Read the model definition and answer for the solid it produces. Units are mm, in the model's axes. A direction names the side the tool comes from. Round coordinates to 2 decimals unless told otherwise and drop trailing zeros. Write each loop counter-clockwise with the first axis right and the second up, starting at its lowest first coordinate (ties: lowest second). Pieces come first, ordered by that corner, then holes. Notation, with made-up numbers: M -3.75,86 L 36.25,86 A26 cw 36.25,113 Z; hole C 34.5,1.25 d2. An arc over 180 degrees is marked long. Use one line per item in the form item = value. Start each with the question number.
```python
from build123d import *

# Parameters (mm, degrees)
BOSS_EXTRUDE1_START         = -15
BOSS_EXTRUDE1_DEPTH         = 30
BOSS_EXTRUDE1_START_2       = -12.7
BOSS_EXTRUDE1_2_OUTLINE_W   = 10
BOSS_EXTRUDE1_2_OUTLINE_H   = 5.949524979
BOSS_EXTRUDE1_2_DEPTH       = 25.4
BOSS_EXTRUDE1_3_OUTLINE_R   = 15
BOSS_EXTRUDE1_3_OUTLINE_R_2 = 4.55
BOSS_EXTRUDE1_3_DEPTH       = 19.994560744
SKETCH4_W                   = 3.6
SKETCH4_H                   = 22.4
CUT_EXTRUDE1_DEPTH          = 6
BOSS_EXTRUDE2_REACH         = 73.536
BOSS_EXTRUDE2_END_RADIUS    = 119.634966004
SKETCH9_R                   = 6.57997386
SKETCH9_R_2                 = 3.45
SKETCH10_W                  = 5.949524979
SKETCH10_H                  = 2.3
BOSS_EXTRUDE3_DEPTH         = 10
SKETCH11_W                  = 5.949524979
SKETCH11_H                  = 30
BOSS_EXTRUDE4_DEPTH         = 10
SKETCH13_W                  = 3.6
SKETCH13_H                  = 22.4
CUT_EXTRUDE2_DEPTH          = 10
CUT_EXTRUDE3_DEPTH          = 5


with BuildPart() as part:
    # Boss-Extrude1: read off the stored shape, not the designer's step
    # Boss-Extrude1 outline → Boss-Extrude1 (new body)
    with BuildSketch(Plane(origin=(0, 0, 0), x_dir=(1, 0, 0), z_dir=(0, 1, 0)).offset(BOSS_EXTRUDE1_START)):
        with BuildLine():
            Line((-50, -30), (-50, -35.949524979))
            ThreePointArc((-50, -35.949524979), (-25.592440765, -27.769436157), (0, -25))
            ThreePointArc((0, -25), (25.592440765, -27.769436157), (50, -35.949524979))
            Line((50, -35.949524979), (50, -30))
            ThreePointArc((50, -30), (27.810549479, -22.327809439), (4.550000287, -19.13702996))
            ThreePointArc((4.550000287, -19.13702996), (2.275411741, -19.072115713), (0, -19.050475021))
            ThreePointArc((0, -19.050475021), (-25.592440765, -21.819911178), (-50, -30))
        make_face()
    extrude(amount=BOSS_EXTRUDE1_DEPTH)

    # Boss-Extrude1 2 outline → Boss-Extrude1 2 (add)
    with BuildSketch(Plane(origin=(0, 0, 0), x_dir=(1, 0, 0), z_dir=(0, 1, 0)).offset(BOSS_EXTRUDE1_START_2)):
        with Locations((-55, -32.97476249)):
            Rectangle(BOSS_EXTRUDE1_2_OUTLINE_W, BOSS_EXTRUDE1_2_OUTLINE_H)
    extrude(amount=BOSS_EXTRUDE1_2_DEPTH)

    # Boss-Extrude1 3 outline → Boss-Extrude1 3 (add)
    with BuildSketch(Plane.XY):
        Circle(BOSS_EXTRUDE1_3_OUTLINE_R)
        Circle(BOSS_EXTRUDE1_3_OUTLINE_R_2, mode=Mode.SUBTRACT)
    extrude(amount=BOSS_EXTRUDE1_3_DEPTH)

    # Sketch4 → Cut-Extrude1 (cut)
    with BuildSketch(Plane.XY.offset(35.949524979)):
        with Locations((-53, 0)):
            Rectangle(SKETCH4_W, SKETCH4_H)
    extrude(amount=-CUT_EXTRUDE1_DEPTH, mode=Mode.SUBTRACT)

    # Boss-Extrude2: up to this cylinder (the profile starts outside it)
    boss_extrude2_end = Plane(origin=(0, 0, 138.685441025), z_dir=(0, -1, 0)) * Cylinder(BOSS_EXTRUDE2_END_RADIUS, 387.341932008, mode=Mode.PRIVATE)
    # Sketch9 → Boss-Extrude2 (add, up to the surface)
    with BuildSketch(Plane(origin=(0, 0, 0), x_dir=(-1, 0, 0), z_dir=(0, 0, -1)), mode=Mode.PRIVATE) as boss_extrude2_sk1:
        Circle(SKETCH9_R)
        Circle(SKETCH9_R_2, mode=Mode.SUBTRACT)
    boss_extrude2_tool1 = extrude(boss_extrude2_sk1.sketch, amount=-BOSS_EXTRUDE2_REACH, mode=Mode.PRIVATE) - boss_extrude2_end
    add(boss_extrude2_tool1.solids().sort_by_distance((6.393864, 0, 0))[0])

    # Sketch10 → Boss-Extrude3 (add)
    with BuildSketch(Plane.ZY.offset(50)):
        with Locations((32.97476249, 13.85)):
            Rectangle(SKETCH10_W, SKETCH10_H)
        with Locations((32.97476249, -13.85)):
            Rectangle(SKETCH10_W, SKETCH10_H)
    extrude(amount=BOSS_EXTRUDE3_DEPTH)

    # Sketch11 → Boss-Extrude4 (add)
    with BuildSketch(Plane(origin=(50, 0, 0), x_dir=(0, 0, -1), z_dir=(1, 0, 0))):
        with Locations((-32.97476249, 0)):
            Rectangle(SKETCH11_W, SKETCH11_H)
    extrude(amount=BOSS_EXTRUDE4_DEPTH)

    # Sketch13 → Cut-Extrude2 (cut)
    with BuildSketch(Plane.XY.offset(35.949524979)):
        with Locations((53, 0)):
            Rectangle(SKETCH13_W, SKETCH13_H)
    extrude(amount=-CUT_EXTRUDE2_DEPTH, mode=Mode.SUBTRACT)

    # Sketch15 → Cut-Extrude3 (cut)
    with BuildSketch(Plane(origin=(0, 0, 0), x_dir=(-1, 0, 0), z_dir=(0, 0, -1))):
        Polygon((0, 5.831237719), (-5.05, 2.915618859), (-5.05, -2.915618859), (0, -5.831237719), (5.05, -2.915618859), (5.05, 2.915618859), align=None)
    extrude(amount=-CUT_EXTRUDE3_DEPTH, mode=Mode.SUBTRACT)


solid = part.part
```
Q1. Find section D-D on y = -8. Write down the section's boundary in (x, z), and give its area (3 significant figures).
Q2. For a pull along X with two mould halves and no side action, classify faces 6 (the face through (56, 0, 35.95)), 7 (the face through (2.49, 4.394, 2.465)), 8 (the face through (60, 0, 33)) as +X half, -X half, draft (parallel to the pull), parting line (faces both ways), or undercut.
Q3. Find section B-B on z = 28.5. Write down the section's boundary in (x, y).
Q4. A tool of negligible diameter and unlimited length cuts with its end or side. For faces 1 (the face through (56, 0, 30)), 2 (the face through (-56, 0, 35.95)), 3 (the face through (-54.8, 0, 33)), 4 (the face through (2.56, -4.353, 2.465)), 5 (the face through (-56, 0, 30)), from which of +Z, -Z, +X, -X, +Y, -Y can it reach the whole face along a straight path? Write none if from no direction.
Q5. Straight lines are drawn through the part: line 1 (Y direction, x = 0, z = 13); line 2 (Y direction, x = 0, z = 3). For each, find the intervals that lie inside material, in ascending order. Write a range as [from, to].
Q6. Find section A-A on y = 0. Write down the section's boundary in (x, z), and give its area (3 significant figures).
Q7. Find section C-C on z = 10.5. Write down the section's boundary in (x, y), and give its area (3 significant figures).
Q8. Each of these flat-tipped pins is pushed along its axis until it touches: pin 1 Ø2 at (y, z) = (2, 10) entering from -X; pin 2 Ø4 at (x, y) = (0, 0) entering from -Z; pin 3 Ø4 at (x, y) = (0.5, -2) entering from +Z. Where does it stop, or does it pass through?
Response:
q1.outline = M -60,30 L -54.8,30 L -54.8,35.95 L -60,35.95 Z; M -51.2,30 L -50,30 A119.63 ccw -12.69,19.73 L -12.69,0 L 12.69,0 L 12.69,19.73 A119.63 ccw 50,30 L 51.2,30 L 51.2,35.95 L 50,35.95 A119.63 cw -50,35.95 L -51.2,35.95 Z; M 54.8,30 L 60,30 L 60,35.95 L 54.8,35.95 Z
q1.area = 1,160 mm²
q2.face_6 = draft
q2.face_7 = undercut
q2.face_8 = +X half
q3.outline = M -46.6,-15 L -28.73,-15 L -28.73,15 L -46.6,15 Z; M 28.73,-15 L 46.6,-15 L 46.6,15 L 28.73,15 Z
q4.face_1 = -Z, +X, +Y, -Y
q4.face_2 = +Z, +X, -X, +Y, -Y
q4.face_3 = +Z, -Z
q4.face_4 = -Z
q4.face_5 = -Z, -X, +Y, -Y
q5.line_1 = [-15, -3.45], [3.45, 15]
q5.line_2 = [-15, -5.83], [5.83, 15]
q6.outline = M -60,30 L -54.8,30 L -54.8,35.95 L -60,35.95 Z; M -51.2,30 L -50,30 A119.63 ccw -15,19.99 L -15,0 L -5.05,0 L -5.05,5 L -3.45,5 L -3.45,19.1 A119.63 ccw 3.45,19.1 L 3.45,5 L 5.05,5 L 5.05,0 L 15,0 L 15,19.99 A119.63 ccw 50,30 L 51.2,30 L 51.2,35.95 L 50,35.95 A119.63 cw -50,35.95 L -51.2,35.95 Z; M 54.8,30 L 60,30 L 60,35.95 L 54.8,35.95 Z
q6.area = 1,100 mm²
q7.outline = C 0,0 d30; hole C 0,0 d6.9
q7.area = 669 mm²
q8.pin_1 = -14.97
q8.pin_2 = 19.05
q8.pin_3 = 25.03
